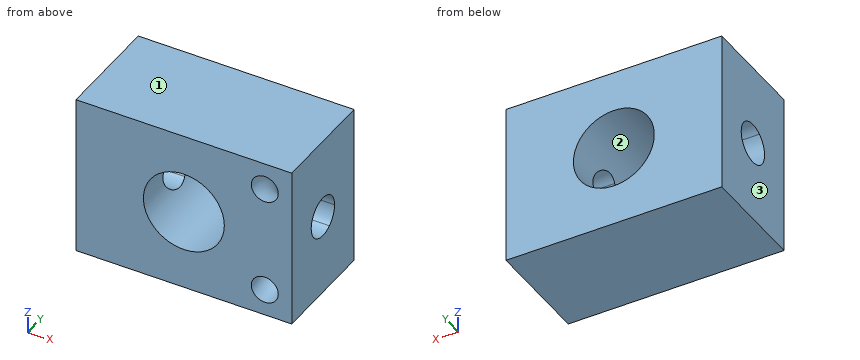
from build123d import *

# Parameters (mm, degrees)
F0_W     = 101.6
F0_H     = 76.2
F1_DEPTH = 50.8
F2_R     = 19.05
F3_DEPTH = 50.801
F5_DEPTH = 101.601
F6_R     = 6.35


with BuildPart() as f1:
    # F0 (on Front) → F1 (new body)
    with BuildSketch(Plane.XZ):
        with Locations((50.8, 38.1)):
            Rectangle(F0_W, F0_H)
    extrude(amount=F1_DEPTH)

    # F2 (on face) → F3 (cut, through all)
    with BuildSketch(Plane.XZ.offset(50.8)):
        with Locations((50.8, 38.1)):
            Circle(F2_R)
    extrude(amount=-F3_DEPTH, mode=Mode.SUBTRACT)

    # F4 (on face) → F5 (cut, through all)
    with BuildSketch(Plane.YZ.offset(101.6)):
        with BuildLine():
            ThreePointArc((-15.875, 38.1), (-20.9055532593, 46.4979505533), (-30.683519369, 46.0252790536))
            Line((-30.683519369, 46.0252790536), (-20.116480631, 30.1747209464))
            ThreePointArc((-20.116480631, 30.1747209464), (-17.0020494467, 33.6055532593), (-15.875, 38.1))
        make_face()
        with BuildLine():
            Line((-20.116480631, 30.1747209464), (-30.683519369, 46.0252790536))
            ThreePointArc((-30.683519369, 46.0252790536), (-33.3252790536, 32.816480631), (-20.116480631, 30.1747209464))
        make_face()
    extrude(amount=-F5_DEPTH, mode=Mode.SUBTRACT)

    # F6 (on face) → F7 (revolve, cut)
    with BuildSketch(Plane.XZ.offset(50.8)):
        with Locations((88.9, 63.5)):
            Circle(F6_R)
    revolve(axis=Axis((91.8411842167, -50.8, 38.1), (-1, 0, 0)), mode=Mode.SUBTRACT)


solid = f1.part
Verification items for the finished model (mm, model axes). Face numbers are marked on the shaded views. Give positions to 0.01 mm unless a question says otherwise; leave off trailing zeros. Order: outer loops, then holes, each group sorted by start corner. A loop starts at its lowest first (then second) coordinate and runs counter-clockwise, first axis right, second up. Notation, with made-up numbers: M 12.5,16.5 L 66.5,16.5 A21 cw 66.5,50.5 Z; hole C 22,18.5 d5. An arc over 180 degrees is marked long. Answer as a JSON object with one key per item and string values. Group by question number.
1) Depth check by flat-ended pin: pin 1 Ø2 at (x, y) = (79, -37) entering from -Z. Enter the tip coordinate at first touch or a pass-through.
2) Cross-section at B-B (y = -5.5). Enter the section's corners in (x, z).
3) Cross-section at D-D (z = 35). Enter the section's corners in (x, y).
4) Scan lines: line 1 along Z through (x, y) = (50.8, -15.5); line 2 along X through (y, z) = (-31, 54); line 3 along Z through (x, y) = (85.5, -43). Record each from-to range of solid material in increasing order. Write a range as [from, to].
5) Mould release check, pull along X, two halves, no side actions. Record for the marked faces 1, 2 and 3: released by +X, released by -X, zero draft, split by the parting line, or undercut.
6) Cross-section at A-A (x = 50.8). Enter the section's corners in (y, z).
7) Cross-section at C-C (x = 76). Enter the section's corners in (y, z) (3 decimals).
Result sheet:
{
 "1": {"pin 1": "stops at z = 0"},
 "2": {"outline": "M 0,0 L 101.6,0 L 101.6,76.2 L 0,76.2 Z; hole C 50.8,38.1 d38.1"},
 "3": {"outline": "M 0,-50.8 L 32,-50.8 L 32,-34.41 L 0,-34.41 Z; M 0,-16.39 L 32,-16.39 L 32,0 L 0,0 Z; M 69.6,-50.8 L 101.6,-50.8 L 101.6,-34.41 L 69.6,-34.41 Z; M 69.6,-16.39 L 101.6,-16.39 L 101.6,0 L 69.6,0 Z"},
 "4": {"line 1": "z = [0, 19.05], [57.15, 76.2]", "line 2": "x = [0, 40.31], [61.29, 82.55], [95.25, 101.6]", "line 3": "z = [0, 8.34], [19.64, 56.56], [67.86, 76.2]"},
 "5": {"face 1": "zero draft", "face 2": "undercut", "face 3": "released by -X"},
 "6": {"outline": "M -50.8,0 L 0,0 L 0,19.05 L -50.8,19.05 Z; M -50.8,57.15 L 0,57.15 L 0,76.2 L -50.8,76.2 Z"},
 "7": {"outline": "M -50.8,0 L 0,0 L 0,76.2 L -50.8,76.2 Z; hole C -25.4,38.1 d19.05"}
}
